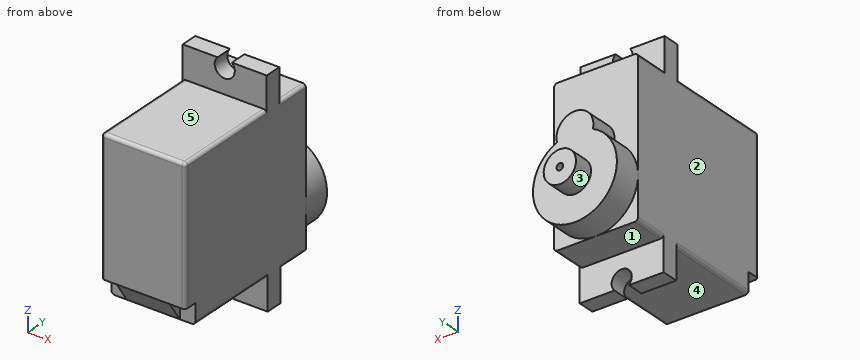
```python
from build123d import *

# Parameters (mm, degrees)
SKETCH1_W               = 12.5
SKETCH1_H               = 23
BOSS_EXTRUDE1_DEPTH     = 24
BOSS_EXTRUDE2_DEPTH     = 4.2
SKETCH3_R               = 2.4
SKETCH3_R_2             = 0.5
BOSS_EXTRUDE3_DEPTH     = 3
SKETCH4_W               = 12.5
SKETCH4_H               = 2.5
BOSS_EXTRUDE4_DEPTH     = 4.75
SKETCH5_W               = 12.5
SKETCH5_H               = 2.5
BOSS_EXTRUDE5_DEPTH     = 4.75
CUT_EXTRUDE1_REACH      = 27.55
SKETCH6_R               = 1.5
CUT_EXTRUDE2_REACH      = 27.697
SKETCH8_R               = 1.5
CUT_EXTRUDE4_DEPTH      = 38.33299479
CUT_EXTRUDE6_DEPTH      = 38.33299479
CUT_EXTRUDE6_DEPTH_BACK = 2.3
CUT_EXTRUDE7_DEPTH      = 38.33299479
CUT_EXTRUDE7_DEPTH_BACK = 2.3
FILLET1_R               = 0.5


with BuildPart() as part:
    # Sketch1 → Boss-Extrude1 (new body)
    with BuildSketch(Plane(origin=(0, 0, 0), x_dir=(1, 0, 0), z_dir=(0, 1, 0))):
        Rectangle(SKETCH1_W, SKETCH1_H)
    extrude(amount=BOSS_EXTRUDE1_DEPTH)

    # Sketch2 → Boss-Extrude2 (add)
    with BuildSketch(Plane(origin=(0, 24, 0), x_dir=(1, 0, 0), z_dir=(0, 1, 0))):
        with BuildLine():
            ThreePointArc((2.682624648, -0.395), (0, 11.5), (-2.682624648, -0.395))
            ThreePointArc((-2.682624648, -0.395), (0, -3.75), (2.682624648, -0.395))
        make_face()
    extrude(amount=BOSS_EXTRUDE2_DEPTH)

    # Sketch3 → Boss-Extrude3 (add)
    with BuildSketch(Plane(origin=(0, 28.2, 0), x_dir=(1, 0, 0), z_dir=(0, 1, 0))):
        with Locations(Location((0, 5.25, 0), (0, 0, 270))):
            Circle(SKETCH3_R)
        with Locations(Location((0, 5.25, 0), (0, 0, 270))):
            Circle(SKETCH3_R_2, mode=Mode.SUBTRACT)
    extrude(amount=BOSS_EXTRUDE3_DEPTH)

    # Sketch4 → Boss-Extrude4 (add)
    with BuildSketch(Plane(origin=(0, 0, -11.5), x_dir=(-1, 0, 0), z_dir=(0, 0, -1))):
        with Locations((0, 17.65)):
            Rectangle(SKETCH4_W, SKETCH4_H)
    extrude(amount=BOSS_EXTRUDE4_DEPTH)

    # Sketch5 → Boss-Extrude5 (add)
    with BuildSketch(Plane.XY.offset(11.5)):
        with Locations((0, 17.45)):
            Rectangle(SKETCH5_W, SKETCH5_H)
    extrude(amount=BOSS_EXTRUDE5_DEPTH)

    # Sketch6 → Cut-Extrude1 (cut, up to next)
    with BuildSketch(Plane(origin=(0, 18.7, 0), x_dir=(1, 0, 0), z_dir=(0, 1, 0)), mode=Mode.PRIVATE) as cut_extrude1_sk1:
        with Locations((0, -15.2)):
            Circle(SKETCH6_R)
    cut_extrude1_tool1 = extrude(cut_extrude1_sk1.sketch, amount=-CUT_EXTRUDE1_REACH, mode=Mode.PRIVATE) & part.part
    add(cut_extrude1_tool1.solids().sort_by_distance((0, 18.7, 15.2))[0], mode=Mode.SUBTRACT)

    # Sketch8 → Cut-Extrude2 (cut, up to next)
    with BuildSketch(Plane(origin=(0, 18.9, 0), x_dir=(1, 0, 0), z_dir=(0, 1, 0)), mode=Mode.PRIVATE) as cut_extrude2_sk1:
        with Locations((0, 15.2)):
            Circle(SKETCH8_R)
    cut_extrude2_tool1 = extrude(cut_extrude2_sk1.sketch, amount=-CUT_EXTRUDE2_REACH, mode=Mode.PRIVATE) & part.part
    add(cut_extrude2_tool1.solids().sort_by_distance((0, 18.9, -15.2))[0], mode=Mode.SUBTRACT)

    # Sketch9 → Cut-Extrude4 (cut, through all)
    with BuildSketch(Plane(origin=(6.25, 0, 0), x_dir=(0, 0, -1), z_dir=(1, 0, 0))):
        Polygon((11.5, 2), (8.5, 0), (11.5, 0), align=None)
    extrude(amount=-CUT_EXTRUDE4_DEPTH, mode=Mode.SUBTRACT)

    # Sketch10 → Cut-Extrude6 (cut, two sides: drawn at the far end of the back side and taken through both)
    with BuildSketch(Plane(origin=(6.25, 0, 0), x_dir=(0, 0, -1), z_dir=(1, 0, 0)).offset(-CUT_EXTRUDE6_DEPTH_BACK)):
        Polygon((102.065563363, 2), (11.5, 2), (8.5, 2), (8.5, 0), (8.5, -90.565563363), (135.889097577, -219.33086493), (229.45466094, -126.765301567), align=None)
    extrude(amount=CUT_EXTRUDE6_DEPTH + CUT_EXTRUDE6_DEPTH_BACK, mode=Mode.SUBTRACT)

    # Sketch11 → Cut-Extrude7 (cut, two sides: drawn at the far end of the back side and taken through both)
    with BuildSketch(Plane.ZY.offset(6.25).offset(-CUT_EXTRUDE7_DEPTH_BACK)):
        Polygon((-102.065563363, 2), (-11.5, 2), (-8.5, 2), (-8.5, 0), (-8.5, -90.565563363), (-135.889097577, -219.33086493), (-229.45466094, -126.765301567), align=None)
    extrude(amount=CUT_EXTRUDE7_DEPTH + CUT_EXTRUDE7_DEPTH_BACK, mode=Mode.SUBTRACT)

    # Fillet1
    fillet1_edges = [part.edges().sort_by_distance(p)[0] for p in [
        (-6.25, 9.2, -11.5),
        (6.25, 9.2, -11.5),
        (6.25, 8.1, 11.5),
        (-6.25, 8.1, 11.5),
        (6.25, 0, 1.5),
        (0, 0, 11.5),
        (-6.25, 21.45, -11.5),
        (6.25, 21.45, -11.5),
        (6.25, 21.35, 11.5),
        (-6.25, 0, 1.5),
        (-6.25, 21.35, 11.5),
    ]]
    fillet(fillet1_edges, radius=FILLET1_R)


solid = part.part
```
Work out the finished part from the listing and answer in its coordinate system (mm). Face numbers are marked on the shaded views. A direction names the side the tool comes from. Give positions to 0.01 mm unless a question says otherwise; leave off trailing zeros. Write each loop counter-clockwise with the first axis right and the second up, starting at its lowest first coordinate (ties: lowest second). Pieces come first, ordered by that corner, then holes.
(1) The part is cut by section A-A on z = -15.2. Write down the section's boundary in (x, y), plus the area to 4 significant figures.
Final values:
outline: (-6.25, 16.4) - (-1.5, 16.4) - (-1.5, 18.9) - (-6.25, 18.9) - close; (1.5, 16.4) - (6.25, 16.4) - (6.25, 18.9) - (1.5, 18.9) - close
area: 23.75 mm2
(2) The part is cut by section B-B on z = 4.5. Write down the section's boundary in (x, y).
Final values:
outline: (-6.25, 0.5) arc R0.5 ccw to (-5.75, 0) - (5.75, 0) arc R0.5 ccw to (6.25, 0.5) - (6.25, 24) - (-6.25, 24) - close
(3) Which of the six approach directions +Z, -Z, +X, -X, +Y, -Y give full straight-line access (tool end or side, diameter ignored) to the marked faces 1, 2, 3, 4 and 5?
Final values:
face 1: -Z, +X, -X, +Y
face 2: +Z, -Z, -X, +Y, -Y
face 3: +Y
face 4: -Z, +X, -X, -Y
face 5: +Z, +X, -X, -Y
(4) The part is cut by section C-C on y = 27. Write down the section's boundary in (x, z) (3 decimals).
Final values:
outline: (-2.683, 0.395) arc R6.25 ccw (long way) to (2.683, 0.395) arc R2.75 ccw (long way) to start
(5) Straight lines are drawn through the part: line 1 (Y direction, x = 1.25, z = -13.5); line 2 (Z direction, x = 4.5, y = 6.5); line 3 (Z direction, x = 0, y = 17.7). For each, find the intervals that lie inside material, in ascending order.
Final values:
line 1: y = 16.4 to 18.9
line 2: z = -11.5 to 11.5
line 3: z = -13.7 to 13.7
(6) Flat-ended cylindrical pins translate along their axes: pin 1 Ø6 at (x, z) = (-1.5, 14) entering from +Y; pin 2 Ø1.6 at (x, y) = (5.5, 0.5) entering from -Z; pin 3 Ø1.9 at (x, z) = (4, -9) entering from +Y. Find the tip coordinate at first contact, or state that the pin passes through.
Final values:
pin 1: stops at y = 24
pin 2: stops at z = -8.5
pin 3: stops at y = 28.2
(7) The part is cut by section D-D on z = 1. Write down the section's boundary in (x, y).
Final values:
outline: (-6.25, 0.5) arc R0.5 ccw to (-5.75, 0) - (5.75, 0) arc R0.5 ccw to (6.25, 0.5) - (6.25, 24) - (2.75, 24) - (2.75, 28.2) - (-2.75, 28.2) - (-2.75, 24) - (-6.25, 24) - close
